```python
from build123d import *

# Parameters (mm, degrees)
F0_W     = 82.7734842896
F0_H     = 163.7785583735
F1_DEPTH = 1
F2_R     = 10
F3_DEPTH = 5
F4_T     = -0.4


with BuildPart() as f1:
    # F0 (on Front) → F1 (new body)
    with BuildSketch(Plane.XZ):
        with Locations((41.3867421448, 81.8892791867)):
            Rectangle(F0_W, F0_H)
    extrude(amount=F1_DEPTH)

    # F2 (on face) → F3 (join)
    with BuildSketch(Plane(origin=(0, 0, 0), x_dir=(-1, 0, 0), z_dir=(0, 1, 0))):
        with Locations((-18.917247653, 23.1196433306)):
            Circle(F2_R)
        with Locations((-18.917247653, 95.850430429)):
            Circle(F2_R)
        with Locations((-41.1302503198, 23.1196433306)):
            Circle(F2_R)
        with Locations((-41.1302503198, 95.850430429)):
            Circle(F2_R)
        with Locations((-63.3432529867, 23.1196433306)):
            Circle(F2_R)
        with Locations((-63.3432529867, 95.850430429)):
            Circle(F2_R)
    extrude(amount=F3_DEPTH)

    # F4
    f4_openings = [f1.faces().sort_by_distance(p)[0] for p in [
        (41.386742, -1, 81.889279),
    ]]
    offset(amount=F4_T, openings=f4_openings, kind=Kind.INTERSECTION)


solid = f1.part
```
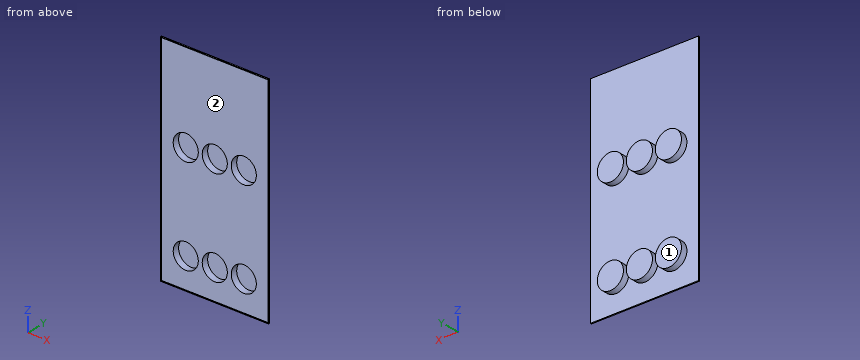
Geometry: final body of the model. Coordinates: model frame, mm. Face numbers are marked on the shaded views. Coordinates: 2 decimals unless noted, no trailing zeros. Order: outer loops, then holes, each group sorted by start corner. A loop starts at its lowest first (then second) coordinate and runs counter-clockwise, first axis right, second up. Notation, with made-up numbers: (44.5, 72) -> (87.5, 72) arc R21 ccw to (87.5, 103) -> close; hole circle Ø2 at (77.5, -11.75). An arc over 180 degrees is marked (long way). Write item = value, one per line.
(1) Pin query (flat end, axial travel): pin 1 Ø1.5 at (y, z) = (1, 73.5) entering from -X; pin 2 Ø11.5 at (x, z) = (41.13, 95.85) entering from -Y; pin 3 Ø4 at (x, z) = (34.5, 76) entering from +Y; pin 4 Ø15.5 at (x, z) = (15, 20) entering from -Y. Return the tip coordinate at first contact, or that it passes through.
Solved:
pin_1 = through
pin_2 = 4.6
pin_3 = 0
pin_4 = -0.4
(2) Cut plane C-C on x = 7. Return loops of the section in (y, z).
Solved:
outline = (-1, 0) -> (0, 0) -> (0, 163.78) -> (-1, 163.78) -> (-1, 163.38) -> (-0.4, 163.38) -> (-0.4, 0.4) -> (-1, 0.4) -> close
(3) Cut plane A-A on z = 65.5. Return loops of the section in (x, y).
Solved:
outline = (0, -1) -> (0.4, -1) -> (0.4, -0.4) -> (82.37, -0.4) -> (82.37, -1) -> (82.77, -1) -> (82.77, 0) -> (0, 0) -> close
(4) Cut plane B-B on y = 3.35. Count the separate pieces of the cut face and the enclosed holes in it, plus the area to 3 significant figures.
Solved:
separate_pieces = 6
enclosed_holes = 6
area = 148 mm²
(5) Pull-direction query (Z, two-part tool) for the marked faces 1 and 2; classes: pulls with the +Z half, pulls with the -Z half, needs draft (parallel to the pull), parting line crosses it, or undercut.
Solved:
face_1 = needs draft
face_2 = undercut
(6) Line query: line 1 (X direction, y = 1.9, z = 23); line 2 (Z direction, x = 11.5, y = 2.5); line 3 (X direction, y = 2.2, z = 92). Output: solid intervals per line, ascending.
Solved:
line_1 = 8.92 to 9.32, 28.52 to 28.92, 31.13 to 31.53, 50.73 to 51.13, 53.34 to 53.74, 72.94 to 73.34
line_2 = 16.41 to 17.03, 29.21 to 29.83, 89.14 to 89.76, 101.95 to 102.56
line_3 = 9.69 to 10.12, 27.71 to 28.15, 31.9 to 32.34, 49.92 to 50.36, 54.11 to 54.55, 72.14 to 72.57
(7) Cut plane D-D on x = 18. Return loops of the section in (y, z), plus the area to 3 significant figures.
Solved:
outline = (-1, 0) -> (0, 0) -> (0, 13.16) -> (5, 13.16) -> (5, 33.08) -> (0, 33.08) -> (0, 85.89) -> (5, 85.89) -> (5, 105.81) -> (0, 105.81) -> (0, 163.78) -> (-1, 163.78) -> (-1, 163.38) -> (-0.4, 163.38) -> (-0.4, 105.41) -> (4.6, 105.41) -> (4.6, 86.29) -> (-0.4, 86.29) -> (-0.4, 32.68) -> (4.6, 32.68) -> (4.6, 13.56) -> (-0.4, 13.56) -> (-0.4, 0.4) -> (-1, 0.4) -> close
area = 74.0 mm²
